Geometry check sheet. Reference: the model listing, model coordinates, mm. A direction names the side the tool comes from. Give positions to 0.01 mm unless a question says otherwise; leave off trailing zeros. Write each loop counter-clockwise with the first axis right and the second up, starting at its lowest first coordinate (ties: lowest second). Pieces come first, ordered by that corner, then holes. Notation, with made-up numbers: (29.25, 13.5) -> (75.25, 13.5) arc R21 ccw to (75.25, 44.5) -> close; hole circle Ø2 at (52, 48). An arc over 180 degrees is marked (long way). Use a Markdown table: item, result. Add a question column.
from build123d import *

# Parameters (mm, degrees)
SKETCH_1_W             = 55
SKETCH_1_H             = 74.5
SKETCH_1_R             = 2.2
SKETCH_1_W_2           = 12
SKETCH_1_H_2           = 3
EXTRUDE_1_DEPTH        = 3
SKETCH_2_W             = 3.3
SKETCH_2_H             = 10.4
CUT_EXTRUDE_1_DEPTH    = 3
SKETCH_3_W             = 1.35
SKETCH_3_H             = 3.3
SKETCH_3_W_2           = 3.3
SKETCH_3_H_2           = 2.7
SKETCH_3_H_3           = 6
CUT_EXTRUDE_2_DEPTH    = 3
PATTERN_LINEAR_1_COUNT = 2
PATTERN_LINEAR_1_PITCH = 25


with BuildPart() as part:
    # 草图1 → 凸台-拉伸1 (new body)
    # profile 1 of 3: a face of its own
    with BuildSketch(Plane(origin=(0, 0, 0), x_dir=(1, 0, 0), z_dir=(0, 1, 0))):
        Rectangle(SKETCH_1_W, SKETCH_1_H)
        with Locations(Location((0, 27.25, 0), (0, 0, 270))):
            Circle(SKETCH_1_R, mode=Mode.SUBTRACT)
        with Locations(Location((-15, 27.25, 0), (0, 0, 270))):
            Circle(SKETCH_1_R, mode=Mode.SUBTRACT)
        with Locations(Location((15, 27.25, 0), (0, 0, 270))):
            Circle(SKETCH_1_R, mode=Mode.SUBTRACT)
    # profile 2 of 3: a face of its own
    with BuildSketch(Plane(origin=(0, 0, 0), x_dir=(1, 0, 0), z_dir=(0, 1, 0))):
        with Locations((-13, -38.75)):
            Rectangle(SKETCH_1_W_2, SKETCH_1_H_2)
    # profile 3 of 3: a face of its own
    with BuildSketch(Plane(origin=(0, 0, 0), x_dir=(1, 0, 0), z_dir=(0, 1, 0))):
        with Locations((13, -38.75)):
            Rectangle(SKETCH_1_W_2, SKETCH_1_H_2)
    extrude(amount=EXTRUDE_1_DEPTH)

    # 草图2 → 切除-拉伸1 (cut)
    with BuildSketch(Plane(origin=(0, 3, 0), x_dir=(1, 0, 0), z_dir=(0, 1, 0))):
        with Locations((-21.85, -20.05)):
            Rectangle(SKETCH_2_W, SKETCH_2_H)
        with Locations((21.85, -20.05)):
            Rectangle(SKETCH_2_W, SKETCH_2_H)
    cut_extrude_1 = extrude(amount=-CUT_EXTRUDE_1_DEPTH, mode=Mode.SUBTRACT)

    # 草图3 → 切除-拉伸2 (cut)
    with BuildSketch(Plane(origin=(0, 3, 0), x_dir=(1, 0, 0), z_dir=(0, 1, 0))):
        with Locations((-10.675, -32.6)):
            Rectangle(SKETCH_3_W, SKETCH_3_H)
        with Locations((-13, -29.6)):
            Rectangle(SKETCH_3_W_2, SKETCH_3_H_2)
        with Locations((-13, -32.6)):
            Rectangle(SKETCH_3_W_2, SKETCH_3_H)
        with Locations((-13, -37.25)):
            Rectangle(SKETCH_3_W_2, SKETCH_3_H_3)
        with Locations((-15.325, -32.6)):
            Rectangle(SKETCH_3_W, SKETCH_3_H)
        with Locations((13, -37.25)):
            Rectangle(SKETCH_3_W_2, SKETCH_3_H_3)
        with Locations((15.325, -32.6)):
            Rectangle(SKETCH_3_W, SKETCH_3_H)
        with Locations((13, -32.6)):
            Rectangle(SKETCH_3_W_2, SKETCH_3_H)
        with Locations((13, -29.6)):
            Rectangle(SKETCH_3_W_2, SKETCH_3_H_2)
        with Locations((10.675, -32.6)):
            Rectangle(SKETCH_3_W, SKETCH_3_H)
    extrude(amount=-CUT_EXTRUDE_2_DEPTH, mode=Mode.SUBTRACT)

    # 阵列(线性)1: 切除-拉伸1 ×2
    with Locations(*[(0, 0, -i * PATTERN_LINEAR_1_PITCH) for i in range(1, PATTERN_LINEAR_1_COUNT)]):
        add(cut_extrude_1, mode=Mode.SUBTRACT)


solid = part.part
1) Sectioned sample at A-A, the plane x = 0. Enter the section's corners in (y, z).
2) Tool access check on faces 4 (the face through (-9, 1, 40.25)), 5 (the face through (22, 2, 25.25)), 6 (the face through (-7, 1, 39)), 7 (the face through (-19, 1, 39)). Record the directions out of +Z, -Z, +X, -X, +Y, -Y that give a thin tool (end or side, any length) a straight path to the whole face; none if there is none.
3) Draft check along X on faces 1 (the face through (11.35, 2, 37)), 2 (the face through (-27.5, 1, 1)), 3 (the face through (17, 1, 40.25)). Enter one of: +X half, -X half, draft (parallel to the pull), parting line (faces both ways), or undercut.
4) Sectioned sample at C-C, the plane x = -21.5. Enter the section's corners in (y, z), and give its area (3 significant figures).
5) Gauge pin test, flat ends, axial feed: P1, Ø2.5, axis at x = 15, z = -27.25, coming from the -Y side; P2, Ø1.5, axis at y = 1.5, z = 38.5, coming from the +X side; P3, Ø0.9, axis at x = 25, y = 2, coming from the +Z side. Record the tip position at first contact, or that the pin passes through.
6) Material ranges on probe 1 along X at (y, z) = (1.5, -27.25); probe 2 along X at (y, z) = (2.1, -5.5); probe 3 along X at (y, z) = (0.8, 36), recorded low to high. Write a range as [from, to].
7) Sectioned sample at B-B, the plane z = -27.25. Enter the section's corners in (x, y).
8) Sectioned sample at D-D, the plane z = -4. Enter the section's corners in (x, y).
Check values:
| question | item | result |
|---|---|---|
| 1 | outline | (0, -37.25) -> (3, -37.25) -> (3, -29.45) -> (0, -29.45) -> close; (0, -25.05) -> (3, -25.05) -> (3, 37.25) -> (0, 37.25) -> close |
| 2 | face 4 | +Z, +X, -X, +Y, -Y |
| 2 | face 5 | +Y, -Y |
| 2 | face 6 | +Z, +Y, -Y |
| 2 | face 7 | +Z, -X, +Y, -Y |
| 3 | face 1 | undercut |
| 3 | face 2 | -X half |
| 3 | face 3 | draft |
| 4 | outline | (0, -37.25) -> (3, -37.25) -> (3, -10.15) -> (0, -10.15) -> close; (0, 0.25) -> (3, 0.25) -> (3, 14.85) -> (0, 14.85) -> close; (0, 25.25) -> (3, 25.25) -> (3, 37.25) -> (0, 37.25) -> close |
| 4 | area | 161 mm² |
| 5 | P1 | through |
| 5 | P2 | x = 19 |
| 5 | P3 | z = 37.25 |
| 6 | probe 1 | [-27.5, -17.2], [-12.8, -2.2], [2.2, 12.8], [17.2, 27.5] |
| 6 | probe 2 | [-27.5, -23.5], [-20.2, 20.2], [23.5, 27.5] |
| 6 | probe 3 | [-27.5, -14.65], [-11.35, 11.35], [14.65, 27.5] |
| 7 | outline | (-27.5, 0) -> (-17.2, 0) -> (-17.2, 3) -> (-27.5, 3) -> close; (-12.8, 0) -> (-2.2, 0) -> (-2.2, 3) -> (-12.8, 3) -> close; (2.2, 0) -> (12.8, 0) -> (12.8, 3) -> (2.2, 3) -> close; (17.2, 0) -> (27.5, 0) -> (27.5, 3) -> (17.2, 3) -> close |
| 8 | outline | (-27.5, 0) -> (-23.5, 0) -> (-23.5, 3) -> (-27.5, 3) -> close; (-20.2, 0) -> (20.2, 0) -> (20.2, 3) -> (-20.2, 3) -> close; (23.5, 0) -> (27.5, 0) -> (27.5, 3) -> (23.5, 3) -> close |
